from build123d import *

# Parameters (mm, degrees)
SKETCH1_R           = 3
SKETCH1_R_2         = 7.5
BOSS_EXTRUDE1_DEPTH = 2.5
FILLET1_R           = 30
FILLET2_R           = 15


with BuildPart() as part:
    # Sketch1 → Boss-Extrude1 (new, symmetric)
    with BuildSketch(Plane(origin=(0, 0, 0), x_dir=(1, 0, 0), z_dir=(0, 1, 0))):
        with BuildLine():
            Line((-79, 94), (79, 94))
            ThreePointArc((79, 94), (89.606601718, 89.606601718), (94, 79))
            Line((94, 79), (94, -79))
            ThreePointArc((94, -79), (89.606601718, -89.606601718), (79, -94))
            Line((79, -94), (-79, -94))
            ThreePointArc((-79, -94), (-89.606601718, -89.606601718), (-94, -79))
            Line((-94, -79), (-94, -30))
            Line((-94, -30), (-154, -30))
            Line((-154, -30), (-154, 30))
            Line((-154, 30), (-94, 30))
            Line((-94, 30), (-94, 79))
            ThreePointArc((-94, 79), (-89.606601718, 89.606601718), (-79, 94))
        make_face()
        with Locations(Location((-76.013978978, 76.013978978, 0), (0, 0, 270))):
            Circle(SKETCH1_R, mode=Mode.SUBTRACT)
        with Locations(Location((76.013978978, 76.013978978, 0), (0, 0, 270))):
            Circle(SKETCH1_R, mode=Mode.SUBTRACT)
        with Locations(Location((76.013978978, -76.013978978, 0), (0, 0, 270))):
            Circle(SKETCH1_R, mode=Mode.SUBTRACT)
        with Locations(Location((-76.013978978, -76.013978978, 0), (0, 0, 270))):
            Circle(SKETCH1_R, mode=Mode.SUBTRACT)
        with Locations(Location((-135, 0, 0), (0, 0, 270))):
            Circle(SKETCH1_R_2, mode=Mode.SUBTRACT)
        with BuildLine():
            Line((29.446798758, -70.384478511), (-29.446798758, -70.384478511))
            ThreePointArc((-29.446798758, -70.384478511), (-31.294557823, -69.149845375), (-30.86101232, -66.970264948))
            Line((-30.86101232, -66.970264948), (-1.414213562, -37.52346619))
            ThreePointArc((-1.414213562, -37.52346619), (0, -36.937679753), (1.414213562, -37.52346619))
            Line((1.414213562, -37.52346619), (30.86101232, -66.970264948))
            ThreePointArc((30.86101232, -66.970264948), (31.294557823, -69.149845375), (29.446798758, -70.384478511))
        make_face(mode=Mode.SUBTRACT)
        with BuildLine():
            Line((-70.384478511, -29.446798758), (-70.384478511, 29.446798758))
            ThreePointArc((-70.384478511, 29.446798758), (-69.149845375, 31.294557823), (-66.970264948, 30.86101232))
            Line((-66.970264948, 30.86101232), (-37.52346619, 1.414213562))
            ThreePointArc((-37.52346619, 1.414213562), (-36.937679753, 0), (-37.52346619, -1.414213562))
            Line((-37.52346619, -1.414213562), (-66.970264948, -30.86101232))
            ThreePointArc((-66.970264948, -30.86101232), (-69.149845375, -31.294557823), (-70.384478511, -29.446798758))
        make_face(mode=Mode.SUBTRACT)
        with BuildLine():
            Line((-29.446798758, 70.384478511), (29.446798758, 70.384478511))
            ThreePointArc((29.446798758, 70.384478511), (31.294557823, 69.149845375), (30.86101232, 66.970264948))
            Line((30.86101232, 66.970264948), (1.414213562, 37.52346619))
            ThreePointArc((1.414213562, 37.52346619), (0, 36.937679753), (-1.414213562, 37.52346619))
            Line((-1.414213562, 37.52346619), (-30.86101232, 66.970264948))
            ThreePointArc((-30.86101232, 66.970264948), (-31.294557823, 69.149845375), (-29.446798758, 70.384478511))
        make_face(mode=Mode.SUBTRACT)
        with BuildLine():
            Line((70.384478511, 29.446798758), (70.384478511, -29.446798758))
            ThreePointArc((70.384478511, -29.446798758), (69.149845375, -31.294557823), (66.970264948, -30.86101232))
            Line((66.970264948, -30.86101232), (37.52346619, -1.414213562))
            ThreePointArc((37.52346619, -1.414213562), (36.937679753, 0), (37.52346619, 1.414213562))
            Line((37.52346619, 1.414213562), (66.970264948, 30.86101232))
            ThreePointArc((66.970264948, 30.86101232), (69.149845375, 31.294557823), (70.384478511, 29.446798758))
        make_face(mode=Mode.SUBTRACT)
    extrude(amount=BOSS_EXTRUDE1_DEPTH, both=True)

    # Fillet1
    fillet1_edges = [part.edges().sort_by_distance(p)[0] for p in [
        (-94, 0, 30),
        (-94, 0, -30),
    ]]
    fillet(fillet1_edges, radius=FILLET1_R)

    # Fillet2
    fillet2_edges = [part.edges().sort_by_distance(p)[0] for p in [
        (-154, 0, 30),
        (-154, 0, -30),
    ]]
    fillet(fillet2_edges, radius=FILLET2_R)


solid = part.part
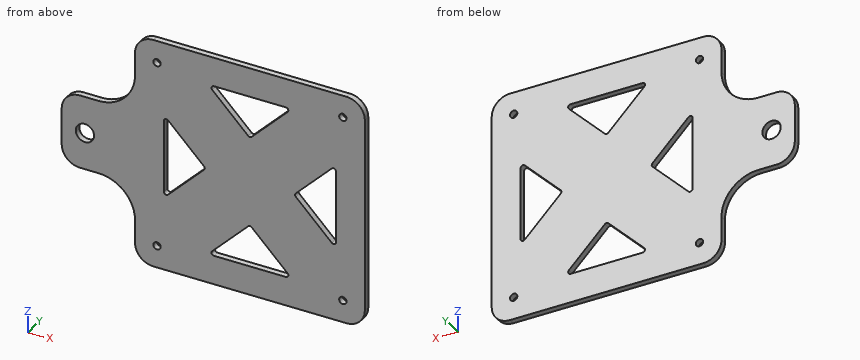
Source: CAD feature listing. Evaluate the final solid. Frame: model axes, mm. Round coordinates to 2 decimals unless told otherwise and drop trailing zeros. Loops run counter-clockwise (first coordinate to the right, second up) from the corner with the lowest first, then second, coordinate; pieces in that order, holes last. Notation, with made-up numbers: M 17.25,-21 L 67.25,-21 A13 ccw 67.25,-2 Z; hole C -36,33.5 d5. An arc over 180 degrees is marked long. Return JSON: item names as keys, results as strings. Group by question number.
1. Material intervals for line 1 along X through (y, z) = (0.1, 0); line 2 along Z through (x, y) = (-30.5, -0.25); line 3 along X through (y, z) = (-0.2, 11.5), sorted ascending. Write a range as from..to.
2. Section query B-B on z = 47. Output: boundary loops of the cut face in (x, y).
3. Section query A-A on x = -135. Output: boundary loops of the cut face in (y, z).
4. Pin query (flat end, axial travel): pin 1 (7 mm diameter, centred on x = -76.01, z = -76.01, fed in from +Y); pin 2 (12 mm diameter, centred on x = -135, z = 0, fed in from -Y). Return the tip coordinate at first contact, or that it passes through.
5. Section query C-C on y = -0.4. State how many separate pieces and enclosed holes the cut face has, and give its area (3 significant figures).
Checks:
{
 "1": {"line 1": "x = -154..-142.5, -127.5..-70.38, -36.94..36.94, 70.38..94", "line 2": "z = -94..-70.08, -66.61..66.61, 70.08..94", "line 3": "x = -154..-70.38, -47.61..47.61, 70.38..94"},
 "2": {"outline": "M -96.96,-2.5 L -10.89,-2.5 L -10.89,2.5 L -96.96,2.5 Z; M 10.89,-2.5 L 94,-2.5 L 94,2.5 L 10.89,2.5 Z"},
 "3": {"outline": "M -2.5,-30 L 2.5,-30 L 2.5,-7.5 L -2.5,-7.5 Z; M -2.5,7.5 L 2.5,7.5 L 2.5,30 L -2.5,30 Z"},
 "4": {"pin 1": "stops at y = 2.5", "pin 2": "passes through"},
 "5": {"separate pieces": "1", "enclosed holes": "9", "area": "34,100 mm²"}
}
